CAD build for the part. Positions are in the model's coordinates, mm. A direction names the side the tool comes from. Coordinates: 2 decimals unless noted, no trailing zeros. Order: outer loops, then holes, each group sorted by start corner. A loop starts at its lowest first (then second) coordinate and runs counter-clockwise, first axis right, second up. Notation, with made-up numbers: (80, 73.25) -> (98, 73.25) arc R7 cw to (98, 85.25) -> close; hole circle Ø9 at (47, 0.25). An arc over 180 degrees is marked (long way). Use one line per item in the form item = value. Start each with the question number.
from build123d import *

# Parameters (mm, degrees)
SKETCH_1_W          = 5
SKETCH_1_H          = 12.5
SKETCH_1_R          = 1.5
EXTRUDE_1_DEPTH     = 8
SKETCH_2_R          = 2.5
CUT_EXTRUDE_1_DEPTH = 10


with BuildPart() as part:
    # 草图1 → 凸台-拉伸1 (new body)
    with BuildSketch(Plane.XY):
        Polygon((2.0625, 31.40625), (-45.9375, 31.40625), (-45.9375, 11.40625), (-55.9375, 11.40625), (-55.9375, -28.59375), (-45.9375, -28.59375), (-45.9375, -48.59375), (2.0625, -48.59375), (2.0625, -28.59375), (12.0625, -28.59375), (12.0625, 11.40625), (2.0625, 11.40625), align=None)
        with Locations((4.5625, 0.15625)):
            Rectangle(SKETCH_1_W, SKETCH_1_H, mode=Mode.SUBTRACT)
        with Locations((4.5625, -17.34375)):
            Rectangle(SKETCH_1_W, SKETCH_1_H, mode=Mode.SUBTRACT)
        with Locations((-39.9375, -43.59375)):
            Circle(SKETCH_1_R, mode=Mode.SUBTRACT)
        with Locations((-39.9375, -19.59375)):
            Circle(SKETCH_1_R, mode=Mode.SUBTRACT)
        with Locations((-48.4375, -17.34375)):
            Rectangle(SKETCH_1_W, SKETCH_1_H, mode=Mode.SUBTRACT)
        with Locations((-3.9375, -43.59375)):
            Circle(SKETCH_1_R, mode=Mode.SUBTRACT)
        with Locations((-3.9375, -19.59375)):
            Circle(SKETCH_1_R, mode=Mode.SUBTRACT)
        with Locations((-48.4375, 0.15625)):
            Rectangle(SKETCH_1_W, SKETCH_1_H, mode=Mode.SUBTRACT)
        with Locations((-39.9375, 2.40625)):
            Circle(SKETCH_1_R, mode=Mode.SUBTRACT)
        with Locations((-39.9375, 26.40625)):
            Circle(SKETCH_1_R, mode=Mode.SUBTRACT)
        with Locations((-3.9375, 2.40625)):
            Circle(SKETCH_1_R, mode=Mode.SUBTRACT)
        with Locations((-3.9375, 26.40625)):
            Circle(SKETCH_1_R, mode=Mode.SUBTRACT)
    extrude(amount=EXTRUDE_1_DEPTH)

    # 草图2 → 切除-拉伸1 (cut)
    with BuildSketch(Plane.XY.offset(8)):
        with Locations((-39.9375, -8.59375)):
            Circle(SKETCH_2_R)
        with Locations((-3.9375, -8.59375)):
            Circle(SKETCH_2_R)
    extrude(amount=-CUT_EXTRUDE_1_DEPTH, mode=Mode.SUBTRACT)


solid = part.part
1) Two-plate mould, pull along Y, no slides. Class faces 4 (the face through (-22, -48.594, 4)), 5 (the face through (-55.938, -8, 4)), 6 (the face through (-48, -6.094, 4)): released by +Y, released by -Y, zero draft, split by the parting line, or undercut.
2) Cut at C-C on x = -4.5. Give the cut face in (y, z), then the cut area to 3 significant figures.
3) 3-axis set-ups, long thin cutter, end or side, ignore diameter. For faces 1 (the face through (5, -11.094, 4)), 2 (the face through (-45.938, -38, 4)), 3 (the face through (-22, -8, 8)): which of +Z, -Z, +X, -X, +Y, -Y reach the whole face in a straight line?
4) Drop flat-ended pins along their axis: P1, Ø1.8, axis at x = -3.94, y = 26.41, coming from the -Z side; P2, Ø1.5, axis at x = -48.5, z = 5.5, coming from the -Y side; P3, Ø4, axis at y = -34.5, z = 3, coming from the -X side; P4, Ø4, axis at x = -48, z = 3.5, coming from the +Y side. Give the stop position or say it passes through.
5) Cut at A-A on x = -50. Give the cut face in (y, z).
6) Cut at D-D on z = 4.25. Count the separate pieces of the cut face and the enclosed holes in it, then the cut area to 3 significant figures.
7) Cut at B-B on y = -22. Give the cut face in (x, z), then the cut area to 3 significant figures.
8) Probe L1, parallel to X at y = -2, z = 0.5; L2, parallel to X at y = -8.5, z = 4.5; L3, parallel to Y at x = 5, z = 6.5. List the from-to ranges inside material, lowest first.
Values follow:
q1.face_4 = released by -Y
q1.face_5 = zero draft
q1.face_6 = undercut
q2.outline = (-48.59, 0) -> (-44.98, 0) -> (-44.98, 8) -> (-48.59, 8) -> close; (-42.2, 0) -> (-20.98, 0) -> (-20.98, 8) -> (-42.2, 8) -> close; (-18.2, 0) -> (-11.03, 0) -> (-11.03, 8) -> (-18.2, 8) -> close; (-6.16, 0) -> (1.02, 0) -> (1.02, 8) -> (-6.16, 8) -> close; (3.8, 0) -> (25.02, 0) -> (25.02, 8) -> (3.8, 8) -> close; (27.8, 0) -> (31.41, 0) -> (31.41, 8) -> (27.8, 8) -> close
q2.area = 512 mm^2
q3.face_1 = +Z, -Z
q3.face_2 = +Z, -Z, -X, -Y
q3.face_3 = +Z, +X, -X, +Y, -Y
q4.P1 = through
q4.P2 = -28.59
q4.P3 = -45.94
q4.P4 = 11.41
q5.outline = (-28.59, 0) -> (-23.59, 0) -> (-23.59, 8) -> (-28.59, 8) -> close; (-11.09, 0) -> (-6.09, 0) -> (-6.09, 8) -> (-11.09, 8) -> close; (6.41, 0) -> (11.41, 0) -> (11.41, 8) -> (6.41, 8) -> close
q6.separate_pieces = 1
q6.enclosed_holes = 14
q6.area = 4,290 mm^2
q7.outline = (-55.94, 0) -> (-50.94, 0) -> (-50.94, 8) -> (-55.94, 8) -> close; (-45.94, 0) -> (2.06, 0) -> (2.06, 8) -> (-45.94, 8) -> close; (7.06, 0) -> (12.06, 0) -> (12.06, 8) -> (7.06, 8) -> close
q7.area = 464 mm^2
q8.L1 = -55.94 to -50.94, -45.94 to 2.06, 7.06 to 12.06
q8.L2 = -55.94 to -42.44, -37.44 to -6.44, -1.44 to 12.06
q8.L3 = -28.59 to -23.59, -11.09 to -6.09, 6.41 to 11.41
